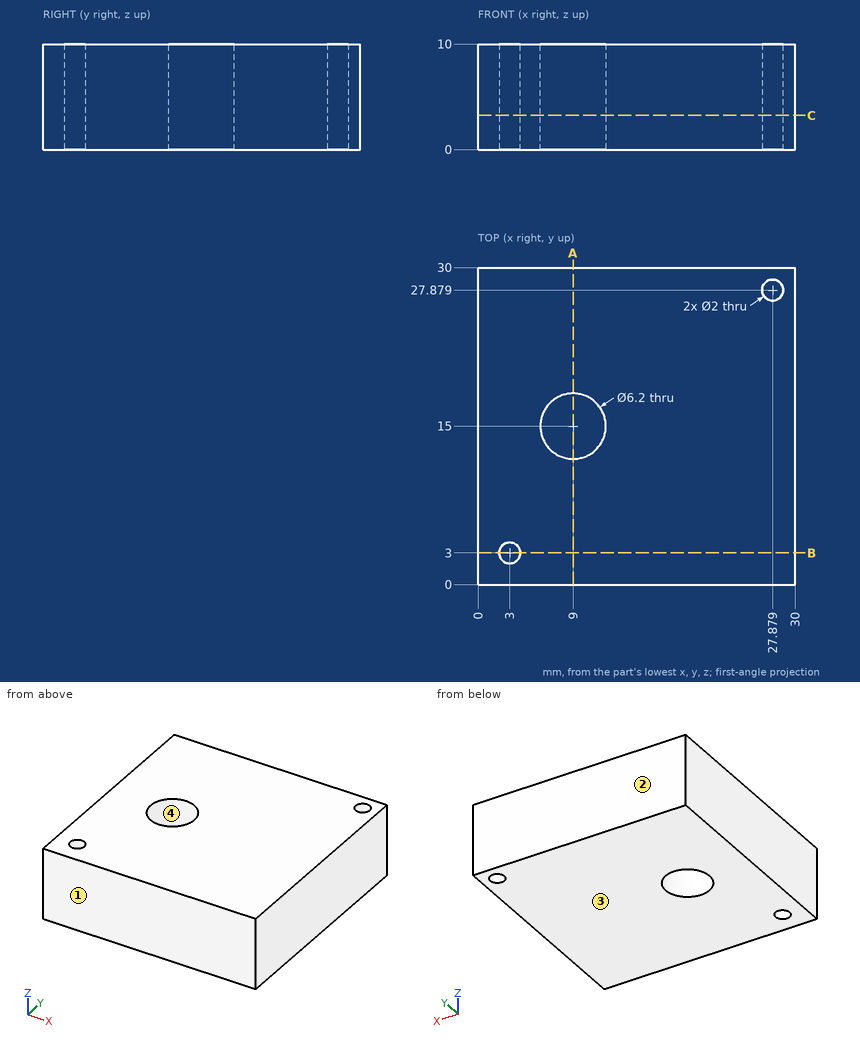
Verification items for this drawing (mm, ordinates from the low corner). Give positions to 0.01 mm unless a question says otherwise; leave off trailing zeros. Loops run counter-clockwise (first coordinate to the right, second up) from the corner with the lowest first, then second, coordinate; pieces in that order, holes last.
(1) Section check B-B on y = 3. Record the cut outline in (x, z), then the cut area to 3 significant figures.
From the geometry:
outline: (0, 0) - (2, 0) - (2, 10) - (0, 10) - close; (4, 0) - (30, 0) - (30, 10) - (4, 10) - close
area: 280 mm2
(2) Thickness scan on L1, parallel to X at y = 3, z = 4; L2, parallel to Y at x = 9, z = 3.25. Record the ranges inside material, lowest first.
From the geometry:
L1: x = 0 to 2, 4 to 30
L2: y = 0 to 11.9, 18.1 to 30
(3) Section check A-A on x = 9. Record the cut outline in (y, z).
From the geometry:
outline: (0, 0) - (11.9, 0) - (11.9, 10) - (0, 10) - close; (18.1, 0) - (30, 0) - (30, 10) - (18.1, 10) - close
(4) Release check for a two-part mould opening along Y. For the marked faces 1, 2, 3 and 4 record: released by +Y, released by -Y, zero draft, split by the parting line, or undercut.
From the geometry:
face 1: released by -Y
face 2: released by +Y
face 3: zero draft
face 4: undercut
(5) Section check C-C on z = 3.25. Record the cut outline in (x, y).
From the geometry:
outline: (0, 0) - (30, 0) - (30, 30) - (0, 30) - close; hole circle Ø2 at (3, 3); hole circle Ø6.2 at (9, 15); hole circle Ø2 at (27.88, 27.88)
